Autodesk Inventor part; units mm, degrees
ref_plane "YZ Plane" through (0, 0, 0) normal (1, 0, 0) x (0, 1, 0)
ref_plane "XZ Plane" through (0, 0, 0) normal (0, 1, 0) x (-1, 0, 0)
ref_plane "XY Plane" through (0, 0, 0) normal (0, 0, 1) x (1, 0, 0)
sketch "Sketch1" plane through (0, 0, 0) normal (0, 0, 1) x (1, 0, 0)
  circle A0 centre (0, 0) radius 3.175
  dimension "d0" = 6.35
extrude "Extrusion1" add sketch "Sketch1" along normal mid plane 101.6
sketch "Sketch2" plane through (0, 0, 50.8) normal (0, 0, 1) x (1, 0, 0)
  circle A0 centre (0, 0) radius 3.175 construction
  circle A1 centre (0, 0) radius 5.7
  dimension "d3" = 11.4
extrude "Extrusion2" add sketch "Sketch2" along normal blind 2
mirror "Mirror1" about plane through (0, 0, 0) normal (0, 0, 1) of "Extrusion2"
properties part number "HINGE PIN" material "Stainless Steel"
Verification items for the finished model (mm, model axes). A direction names the side the tool comes from. Round coordinates to 2 decimals unless told otherwise and drop trailing zeros. Order: outer loops, then holes, each group sorted by start corner. A loop starts at its lowest first (then second) coordinate and runs counter-clockwise, first axis right, second up. Notation, with made-up numbers: (-5, -30) -> (14, -30) arc R23 cw to (14, 7) -> close; hole circle Ø8 at (10, 44). An arc over 180 degrees is marked (long way). Put each result on its own line as item: value.
1) Material ranges on line 1 (Z direction, x = 1.75, y = 5); line 2 (Y direction, x = 0, z = 22) (3 decimals); line 3 (Y direction, x = -1.5, z = 19), recorded low to high.
Final values:
line 1: z = -52.8 to -50.8, 50.8 to 52.8
line 2: y = -3.175 to 3.175
line 3: y = -2.8 to 2.8
2) Mould release check, pull along Z, two halves, no side actions. Record for faces 3 (the flat face through (0, 0, 52.8)), 4 (the flat face through (-2.5, -2.5, -50.8)), 5 (the cylindrical face through (-4.5, 3.5, 51.8)): +Z half, -Z half, draft (parallel to the pull), parting line (faces both ways), or undercut.
Final values:
face 3: +Z half
face 4: undercut
face 5: draft
3) Section check B-B (x = 0). Record the cut outline in (y, z) (3 decimals), then the cut area to 3 significant figures.
Final values:
outline: (-5.7, -52.8) -> (5.7, -52.8) -> (5.7, -50.8) -> (3.175, -50.8) -> (3.175, 50.8) -> (5.7, 50.8) -> (5.7, 52.8) -> (-5.7, 52.8) -> (-5.7, 50.8) -> (-3.175, 50.8) -> (-3.175, -50.8) -> (-5.7, -50.8) -> close
area: 691 mm^2
4) Depth check by flat-ended pin: pin 1 (4 mm diameter, centred on x = 1.5, z = 16.5, fed in from -Y) (3 decimals); pin 2 (3 mm diameter, centred on x = 2, z = 9, fed in from +Y); pin 3 (6 mm diameter, centred on y = 4, z = -15, fed in from -X). Enter the tip coordinate at first touch or a pass-through.
Final values:
pin 1: stops at y = -3.175
pin 2: stops at y = 3.14
pin 3: stops at x = -3.01
5) Set-up check for faces 1 (the flat face through (2.5, -2.5, 50.8)), 2 (the flat face through (0, 0, -52.8)): record each of +Z, -Z, +X, -X, +Y, -Y from which the full face is reachable in a straight line by a thin tool's end or side.
Final values:
face 1: none
face 2: -Z, +X, -X, +Y, -Y
6) Section check C-C (z = 16). Record the cut outline in (x, y) (3 decimals).
Final values:
outline: circle Ø6.35 at (0, 0)
7) Section check A-A (y = 4.25). Record the cut outline in (x, z), then the cut area to 3 significant figures.
Final values:
outline: (-3.8, -52.8) -> (3.8, -52.8) -> (3.8, -50.8) -> (-3.8, -50.8) -> close; (-3.8, 50.8) -> (3.8, 50.8) -> (3.8, 52.8) -> (-3.8, 52.8) -> close
area: 30.4 mm^2
